Autodesk Inventor part; units mm, degrees
ref_plane "YZ Plane" through (0, 0, 0) normal (1, 0, 0) x (0, 1, 0)
ref_plane "XZ Plane" through (0, 0, 0) normal (0, 1, 0) x (-1, 0, 0)
ref_plane "XY Plane" through (0, 0, 0) normal (0, 0, 1) x (1, 0, 0)
sketch "Sketch1" plane through (0, 0, 0) normal (0, 0, 1) x (1, 0, 0)
  line L0 (0, 0) -> (50.8, 0)
  line L1 (50.8, 0) -> (50.8, 25.4)
  line L2 (50.8, 25.4) -> (0, 25.4)
  line L3 (0, 25.4) -> (0, 0)
  dimension "d0" = 50.8
  dimension "d1" = 25.4
extrude "Extrusion1" add sketch "Sketch1" along normal blind 203.2
shell "Shell1" thickness 1.5875 removed faces 2 at (16.9333, 8.4667, 0) at (16.9333, 8.4667, 203.2)
sketch "Sketch2" plane through (0, 25.4, 0) normal (0, 1, 0) x (1, 0, 0)
  circle A0 centre (25.4, -44.45) radius 14.2875
  line L0 (0, 0) -> (0, -203.2)
  line L1 (50.8, 0) -> (0, 0)
  dimension "d5" = 25.4
  dimension "d6" = 44.45
  dimension "d7" = 28.575
extrude "Extrusion2" cut sketch "Sketch2" against normal through all
equation "\"d2\" = Length"
equation "\"Length\" = 203.2"
properties part number "wrist bar boxtube"
Can you work these out from the model? Positions are in its coordinate system, mm. A direction names the side the tool comes from. Give positions to 0.01 mm unless a question says otherwise; leave off trailing zeros. Order: outer loops, then holes, each group sorted by start corner. A loop starts at its lowest first (then second) coordinate and runs counter-clockwise, first axis right, second up. Notation, with made-up numbers: (-32.75, -24.75) - (-17.75, -24.75) arc R19 cw to (-17.75, 7.25) - close; hole circle Ø3 at (61, -25). An arc over 180 degrees is marked (long way). Use a Markdown table: item, result. Add a question column.
Q1. I'm going to push a flat-ended pin straight in: pin 1 (2 mm diameter, centred on y = 19.5, z = 95, fed in from -X). Where does the tip first touch, or does it pass through?
Q2. If we mould it in two halves opening along Y, with no side actions, what happens to faces 1 (the flat face through (25, 1.588, 100)), 2 (the flat face through (49.212, 13, 100)), 3 (the flat face through (0, 13, 100)), 4 (the flat face through (26, 25.4, 100))? For each: released by +Y, released by -Y, zero draft, split by the parting line, or undercut.
Q3. If we section it at D-D on x = 45: Write out the boundary of the cut face in (y, z).
Q4. Please list where these lines run through material, in increasing order: line 1 along X through (y, z) = (20.5, 89.5); line 2 along Y through (x, z) = (14, 31); line 3 along Z through (x, y) = (25.4, 1.1).
Q5. If we section it at B-B on z = 44.45: Write out the boundary of the cut face in (x, y), plus the area to 3 significant figures.
Q6. If we section it at C-C on y = 13.25: Write out the boundary of the cut face in (x, z), plus the area to 3 significant figures.
Q7. On a 3-axis mill with a long thin cutter (end or side, diameter ignored), from which of +Z, -Z, +X, -X, +Y, -Y can I reach the whole of each face in a straight line? I mean faces 5 (the flat face through (26, 23.812, 100)), 6 (the cylindrical face through (14.87, 0.805, 34.794)). Say none if no direction works.
Q8. If we section it at A-A on x = 25.4: Write out the boundary of the cut face in (y, z), plus the area to 3 significant figures.
Answers follow:
| question | item | result |
|---|---|---|
| 1 | pin 1 | stops at x = 0 |
| 2 | face 1 | undercut |
| 2 | face 2 | undercut |
| 2 | face 3 | zero draft |
| 2 | face 4 | released by +Y |
| 3 | outline | (0, 0) - (1.59, 0) - (1.59, 203.2) - (0, 203.2) - close; (23.81, 0) - (25.4, 0) - (25.4, 203.2) - (23.81, 203.2) - close |
| 4 | line 1 | x = 0 to 1.59, 49.21 to 50.8 |
| 4 | line 2 | y = 0 to 1.59, 23.81 to 25.4 |
| 4 | line 3 | z = 0 to 30.16, 58.74 to 203.2 |
| 5 | outline | (0, 0) - (11.11, 0) - (11.11, 1.59) - (1.59, 1.59) - (1.59, 23.81) - (11.11, 23.81) - (11.11, 25.4) - (0, 25.4) - close; (39.69, 0) - (50.8, 0) - (50.8, 25.4) - (39.69, 25.4) - (39.69, 23.81) - (49.21, 23.81) - (49.21, 1.59) - (39.69, 1.59) - close |
| 5 | area | 141 mm^2 |
| 6 | outline | (0, 0) - (1.59, 0) - (1.59, 203.2) - (0, 203.2) - close; (49.21, 0) - (50.8, 0) - (50.8, 203.2) - (49.21, 203.2) - close |
| 6 | area | 645 mm^2 |
| 7 | face 5 | +Z, -Z |
| 7 | face 6 | +Y, -Y |
| 8 | outline | (0, 0) - (1.59, 0) - (1.59, 30.16) - (0, 30.16) - close; (0, 58.74) - (1.59, 58.74) - (1.59, 203.2) - (0, 203.2) - close; (23.81, 0) - (25.4, 0) - (25.4, 30.16) - (23.81, 30.16) - close; (23.81, 58.74) - (25.4, 58.74) - (25.4, 203.2) - (23.81, 203.2) - close |
| 8 | area | 554 mm^2 |
